Autodesk Inventor part; units mm, degrees
ref_plane "YZ Plane" through (0, 0, 0) normal (1, 0, 0) x (0, 1, 0)
ref_plane "XZ Plane" through (0, 0, 0) normal (0, 1, 0) x (-1, 0, 0)
ref_plane "XY Plane" through (0, 0, 0) normal (0, 0, 1) x (1, 0, 0)
sketch "Sketch1" plane through (0, 0, 0) normal (0, 1, 0) x (-1, 0, 0)
  line L0 (0, 0) -> (53, 0)
  line L1 (53, 0) -> (53, -25)
  line L2 (53, -25) -> (0, -25)
  line L3 (0, -25) -> (0, 0)
  circle A0 centre (49, -18) radius 1
  circle A1 centre (49, -7) radius 1
  line L4 (53, -12.5) -> (0, -12.5)
  line L5 (26.5, 0) -> (26.5, -25)
  circle A2 centre (2, -18) radius 1
  circle A3 centre (2, -7) radius 1
  dimension "d228" = 25
  dimension "d229" = 53
  dimension "d232" = 11
  dimension "d233" = 4
  dimension "d234" = 2
  dimension "d240" = 2
extrude "Extrusion1" add sketch "Sketch1" against normal blind 4
properties part number "Langbektang houder"
The listing builds one solid part. Answer for the finished solid, in the listing's coordinates (mm). Coordinates: 2 decimals unless noted, no trailing zeros. Write each loop counter-clockwise with the first axis right and the second up, starting at its lowest first coordinate (ties: lowest second). Pieces come first, ordered by that corner, then holes. Notation, with made-up numbers: M 33,-4 L 59,-4 A12 cw 59,17 Z; hole C -30,67 d11. An arc over 180 degrees is marked long. Use a Markdown table: item, result. Add a question column.
1. Section A-A (x = -49) is taken. Give the vertices of the cut face in (y, z).
2. Section B-B (z = -18) is taken. Give the vertices of the cut face in (x, y).
3. A straight line is drawn through the part: line 1 along Z through (x, y) = (-2, -1.7). Find the intervals that lie inside material, in ascending order. Write a range as [from, to].
4. For a pull along X with two mould halves and no side action, classify faces 1 (the cylindrical face through (-50, -2, -7)), 2 (the cylindrical face through (-2, -2, -19)), 3 (the flat face through (-26, 0, -12)), 4 (the flat face through (0, -2, -13)) as +X half, -X half, draft (parallel to the pull), parting line (faces both ways), or undercut.
Data:
| question | item | result |
|---|---|---|
| 1 | outline | M -4,-25 L 0,-25 L 0,-19 L -4,-19 Z; M -4,-17 L 0,-17 L 0,-8 L -4,-8 Z; M -4,-6 L 0,-6 L 0,0 L -4,0 Z |
| 2 | outline | M -53,-4 L -50,-4 L -50,0 L -53,0 Z; M -48,-4 L -3,-4 L -3,0 L -48,0 Z; M -1,-4 L 0,-4 L 0,0 L -1,0 Z |
| 3 | line 1 | z = [-25, -19], [-17, -8], [-6, 0] |
| 4 | face 1 | undercut |
| 4 | face 2 | undercut |
| 4 | face 3 | draft |
| 4 | face 4 | +X half |
